CAD build for the part. Positions are in the model's coordinates, mm. A direction names the side the tool comes from. Round coordinates to 2 decimals unless told otherwise and drop trailing zeros. Loops run counter-clockwise (first coordinate to the right, second up) from the corner with the lowest first, then second, coordinate; pieces in that order, holes last. Notation, with made-up numbers: M -12.75,9.5 L 22.25,9.5 A20 ccw 22.25,26.5 Z; hole C 38,31 d8. An arc over 180 degrees is marked long. Use one line per item in the form item = value.
from build123d import *

# Parameters (mm, degrees)
SKETCH_2_R          = 2.5
EXTRUDE_1_DEPTH     = 11
CUT_EXTRUDE_1_DEPTH = 5


with BuildPart() as part:
    # 草图2 → 凸台-拉伸1 (new, symmetric)
    with BuildSketch(Plane.XY):
        with BuildLine():
            Line((44.052861038, 4), (34.052861038, 4))
            Line((34.052861038, 4), (34.052861038, 25))
            ThreePointArc((34.052861038, 25), (39.052861038, 30), (44.052861038, 25))
            Line((44.052861038, 25), (44.052861038, 4))
        make_face()
        with Locations((39.052861038, 25)):
            Circle(SKETCH_2_R, mode=Mode.SUBTRACT)
    extrude_1 = extrude(amount=EXTRUDE_1_DEPTH, both=True)

    # 草图3 → 旋转2 (revolve)
    with BuildSketch(Plane.XY, mode=Mode.PRIVATE) as revolve_2_sk:
        with BuildLine():
            Line((29.052861038, 4), (49.052861038, 4))
            Line((49.052861038, 4), (49.052861038, 9))
            ThreePointArc((49.052861038, 9), (47.588394944, 12.535533906), (44.052861038, 14))
            Line((44.052861038, 14), (34.052861038, 14))
            ThreePointArc((34.052861038, 14), (30.517327132, 12.535533906), (29.052861038, 9))
            Line((29.052861038, 9), (29.052861038, 4))
        make_face()
    revolve(revolve_2_sk.sketch.rotate(Axis((27.632077349, 0, 0), (1, 0, 0)), 90), axis=Axis((27.632077349, 0, 0), (1, 0, 0)))

    # 草图4 → 切除-拉伸1 (cut, symmetric)
    with BuildSketch(Plane.XY):
        with BuildLine():
            Line((44.052861038, 15), (44.052861038, 25))
            ThreePointArc((44.052861038, 25), (39.052861038, 30), (34.052861038, 25))
            Line((34.052861038, 25), (34.052861038, 15))
            Line((34.052861038, 15), (44.052861038, 15))
        make_face()
    cut_extrude_1 = extrude(amount=CUT_EXTRUDE_1_DEPTH, both=True, mode=Mode.SUBTRACT)

    # 镜向3: 凸台-拉伸1, 切除-拉伸1 across plane
    add(extrude_1.mirror(Plane.ZX))
    add(cut_extrude_1.mirror(Plane.ZX), mode=Mode.SUBTRACT)


solid = part.part
1. Drop flat-ended pins along their axis: P1, Ø6.5, axis at x = 39.05, y = -25, coming from the +Z side; P2, Ø10, axis at y = 12.5, z = 6, coming from the -X side; P3, Ø2, axis at x = 33, z = 7, coming from the +Y side; P4, Ø5, axis at y = 19.5, z = 4, coming from the -X side. Give the stop position or say it passes through.
Completed:
P1 = 11
P2 = 29.05
P3 = 12.56
P4 = 34.05
2. Pull direction Y, two halves, no side cores. Call faces 1 (the face through (39, 30, -8)), 2 (the face through (39.193, 3.905, -0.867)), 3 (the face through (39, 21, 5)): +Y half, -Y half, draft (parallel to the pull), parting line (faces both ways), or undercut.
Completed:
face_1 = +Y half
face_2 = undercut
face_3 = draft
3. Cut at A-A on y = 17. Write the cut outline in (x, z), and give its area (3 significant figures).
Completed:
outline = M 34.05,-11 L 44.05,-11 L 44.05,-5 L 34.05,-5 Z; M 34.05,5 L 44.05,5 L 44.05,11 L 34.05,11 Z
area = 120 mm2
4. Cut at C-C on y = 0. Write the cut outline in (x, z).
Completed:
outline = M 29.05,-9 A5 ccw 34.05,-14 L 44.05,-14 A5 ccw 49.05,-9 L 49.05,-4 L 29.05,-4 Z; M 29.05,4 L 49.05,4 L 49.05,9 A5 ccw 44.05,14 L 34.05,14 A5 ccw 29.05,9 Z
5. Cut at B-B on y = -26. Write the cut outline in (x, z).
Completed:
outline = M 34.15,-11 L 36.76,-11 L 36.76,-5 L 34.15,-5 Z; M 34.15,5 L 36.76,5 L 36.76,11 L 34.15,11 Z; M 41.34,-11 L 43.95,-11 L 43.95,-5 L 41.34,-5 Z; M 41.34,5 L 43.95,5 L 43.95,11 L 41.34,11 Z
6. Tool access for faces 4 (the face through (39, 17, -11)), 5 (the face through (39, -17, 11)), 6 (the face through (39, -17, -11)), 7 (the face through (39, 21, -5)), 8 (the face through (39, -21, 5)): list every direction of +Z, -Z, +X, -X, +Y, -Y with a clear straight run to the whole face (end or side of a thin tool).
Completed:
face_4 = -Z, +X, -X, +Y
face_5 = +Z, +X, -X, -Y
face_6 = -Z, +X, -X, -Y
face_7 = +X, -X, +Y
face_8 = +X, -X, -Y
7. Probe line 1 along Y through (x, z) = (38.75, 0); line 2 along Z through (x, y) = (40.25, 19.5); line 3 along X through (y, z) = (25, -8.4). List the from-to ranges inside material, lowest first. Write a range as from..to.
Completed:
line_1 = -15..-4, 4..15
line_2 = -11..-5, 5..11
line_3 = 34.05..36.55, 41.55..44.05
8. Cut at D-D on x = 30.5. Write the cut outline in (y, z), and give its area (3 significant figures).
Completed:
outline = C 0,0 d25.04; hole C 0,0 d8
area = 442 mm2
